Check sheet for the modelled part. Datum: model origin and axes. Units: mm. A direction names the side the tool comes from. Round coordinates to 2 decimals unless told otherwise and drop trailing zeros. Write each loop counter-clockwise with the first axis right and the second up, starting at its lowest first coordinate (ties: lowest second). Pieces come first, ordered by that corner, then holes. Notation, with made-up numbers: (69.25, 89) -> (103.25, 89) arc R29 ccw to (103.25, 127) -> close; hole circle Ø8 at (41.5, -5). An arc over 180 degrees is marked (long way). One line per item, written item: value.
Autodesk Inventor part; units mm, degrees
ref_plane "YZ Plane" through (0, 0, 0) normal (1, 0, 0) x (0, 1, 0)
ref_plane "XZ Plane" through (0, 0, 0) normal (0, 1, 0) x (-1, 0, 0)
ref_plane "XY Plane" through (0, 0, 0) normal (0, 0, 1) x (1, 0, 0)
sketch "Sketch1" plane through (0, 0, 0) normal (1, 0, 0) x (0, 1, 0)
  line L0 (-10.25, 27.75) -> (10.25, 27.75)
  line L1 (10.25, 27.75) -> (10.25, -27.75)
  line L2 (10.25, -27.75) -> (-10.25, -27.75)
  line L3 (-10.25, -27.75) -> (-10.25, 27.75)
  line L4 (-10.25, 27.75) -> (10.25, -27.75) construction
  line L5 (10.25, 27.75) -> (-10.25, -27.75) construction
  circle A0 centre (0, 15) radius 2.1
  circle A1 centre (0, -15) radius 2.1
  point P0 (0, 0)
  dimension "d0" = 20.5
  dimension "d1" = 55.5
  dimension "d2" = 4.2
  dimension "d3" = 4.2
  dimension "d4" = 30
  dimension "d5" = 10.25
  dimension "d6" = 12.75
  dimension "d7" = 10.25
extrude "Extrusion1" add sketch "Sketch1" along normal blind 6
sketch "Sketch2" plane through (0, 0, 0) normal (-1, 0, 0) x (0, 0, 1)
  line L0 (27.75, -10.25) -> (-27.75, -10.25)
  line L1 (-27.75, -10.25) -> (-21.75, -10.25)
  line L2 (-21.75, -10.25) -> (-21.75, 10.25)
  line L3 (-21.75, 10.25) -> (-27.75, 10.25)
  line L4 (-27.75, 10.25) -> (-27.75, -10.25)
  line L5 (-27.75, 10.25) -> (27.75, 10.25)
  line L6 (27.75, 10.25) -> (21.75, 10.25)
  line L7 (21.75, 10.25) -> (21.75, -10.25)
  line L8 (21.75, -10.25) -> (27.75, -10.25)
  line L9 (27.75, -10.25) -> (27.75, 10.25)
  point P0 (0, 0)
  dimension "d10" = 6
  dimension "d11" = 20.5
  dimension "d12" = 6
  dimension "d13" = 20.5
extrude "Extrusion2" add sketch "Sketch2" along normal blind 20 contours L0 L7 L5 L9 | L0 L4 L3 L2
sketch "Sketch3" plane through (6, -10.25, 27.75) normal (0, 0, 1) x (1, 0, 0)
  circle A0 centre (-15, 10.25) radius 2.1
  line L0 (0, 20.5) -> (0, 0)
  line L1 (-26, 0) -> (0, 0)
  point P0 (-6, 10.25)
  dimension "d16" = 4.2
  dimension "d17" = 15
  dimension "d18" = 10.25
extrude "Extrusion3" cut sketch "Sketch3" against normal blind 56.5125
properties part number "Bracket Sides" material "Aluminum 6061"
Item 1: Release check for a two-part mould opening along Y. For faces 1 (the cylindrical face through (-11.1, 0.09, -24.71)), 2 (the flat face through (-20, 0, -25)), 3 (the flat face through (1, 10.25, 0)) record: pulls with the +Y half, pulls with the -Y half, needs draft (parallel to the pull), parting line crosses it, or undercut.
Result set:
face 1: undercut
face 2: needs draft
face 3: pulls with the +Y half
Item 2: Sectioned sample at A-A (y = 0). Enter the section's corners in (x, z).
Result set:
outline: (-20, -27.75) -> (-11.1, -27.75) -> (-11.1, -21.75) -> (-20, -21.75) -> close; (-20, 21.75) -> (-11.1, 21.75) -> (-11.1, 27.75) -> (-20, 27.75) -> close; (-6.9, -27.75) -> (6, -27.75) -> (6, -17.1) -> (0, -17.1) -> (0, -21.75) -> (-6.9, -21.75) -> close; (-6.9, 21.75) -> (0, 21.75) -> (0, 17.1) -> (6, 17.1) -> (6, 27.75) -> (-6.9, 27.75) -> close; (0, -12.9) -> (6, -12.9) -> (6, 12.9) -> (0, 12.9) -> close
Item 3: Tool access check on faces 4 (the flat face through (-12, 0, -21.75)), 5 (the cylindrical face through (2.958, -0.273, 12.918)). Record the directions out of +Z, -Z, +X, -X, +Y, -Y that give a thin tool (end or side, any length) a straight path to the whole face; none if there is none.
Result set:
face 4: -X, +Y, -Y
face 5: +X, -X
Item 4: Depth check by flat-ended pin: pin 1 (5 mm diameter, centred on y = 8, z = -5, fed in from -X); pin 2 (6.5 mm diameter, centred on y = 0, z = -15, fed in from +X). Enter the tip coordinate at first touch or a pass-through.
Result set:
pin 1: x = 0
pin 2: x = 6
Item 5: Sectioned sample at D-D (x = -9). Enter the section's corners in (y, z).
Result set:
outline: (-10.25, -27.75) -> (-2.1, -27.75) -> (-2.1, -21.75) -> (-10.25, -21.75) -> close; (-10.25, 21.75) -> (-2.1, 21.75) -> (-2.1, 27.75) -> (-10.25, 27.75) -> close; (2.1, -27.75) -> (10.25, -27.75) -> (10.25, -21.75) -> (2.1, -21.75) -> close; (2.1, 21.75) -> (10.25, 21.75) -> (10.25, 27.75) -> (2.1, 27.75) -> close
Item 6: Material ranges on line 1 along Z through (x, y) = (4.6, 0); line 2 along Y through (x, z) = (-9, -23.1); line 3 along Z through (x, y) = (-15.5, 7), recorded low to high.
Result set:
line 1: -27.75 to -17.1, -12.9 to 12.9, 17.1 to 27.75
line 2: -10.25 to -2.1, 2.1 to 10.25
line 3: -27.75 to -21.75, 21.75 to 27.75
Item 7: Sectioned sample at C-C (z = 15). Enter the section's corners in (x, y).
Result set:
outline: (0, -10.25) -> (6, -10.25) -> (6, -2.1) -> (0, -2.1) -> close; (0, 2.1) -> (6, 2.1) -> (6, 10.25) -> (0, 10.25) -> close
Item 8: Sectioned sample at B-B (x = -5). Enter the section's corners in (y, z).
Result set:
outline: (-10.25, -27.75) -> (10.25, -27.75) -> (10.25, -21.75) -> (-10.25, -21.75) -> close; (-10.25, 21.75) -> (10.25, 21.75) -> (10.25, 27.75) -> (-10.25, 27.75) -> close
